Verification items for this drawing (mm, ordinates from the low corner). A direction names the side the tool comes from. Round coordinates to 2 decimals unless told otherwise and drop trailing zeros. Loops run counter-clockwise (first coordinate to the right, second up) from the corner with the lowest first, then second, coordinate; pieces in that order, holes last. Notation, with made-up numbers: (70, 27) - (101, 27) arc R7 ccw to (101, 40) - close; hole circle Ø5 at (71, 12.25). An arc over 180 degrees is marked (long way). Put each result on its own line as item: value.
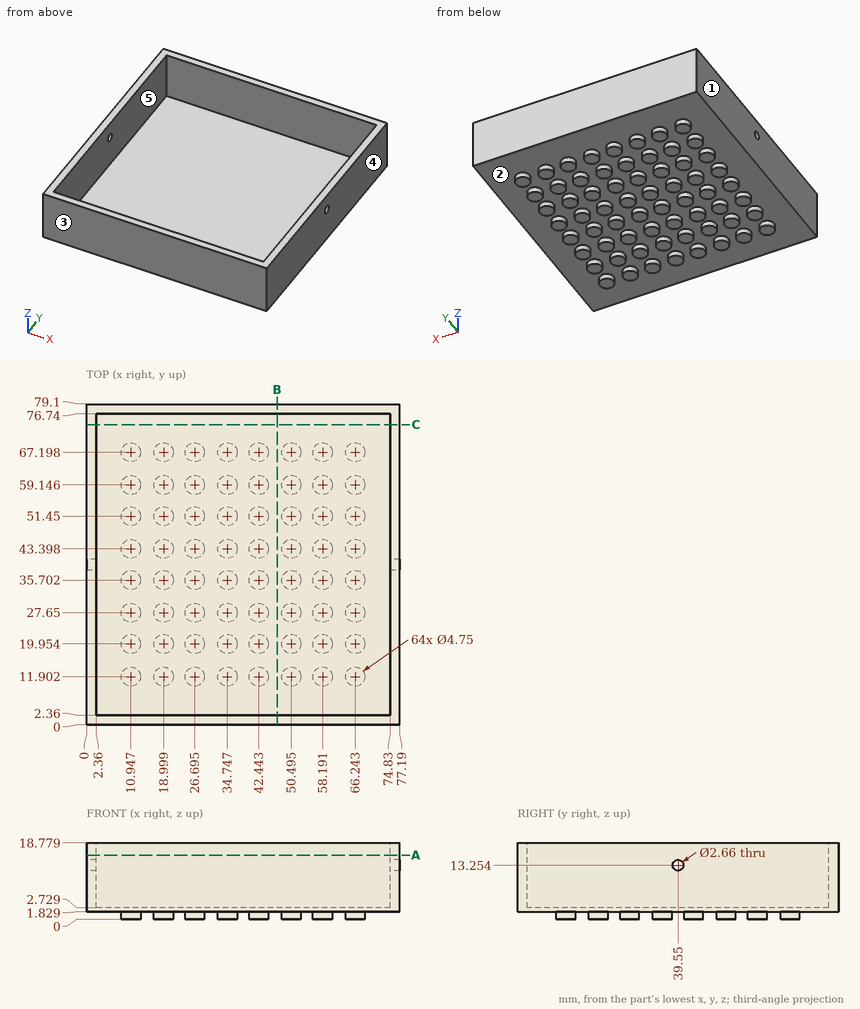
Item 1: Thickness scan on line 1 (Y direction, x = 28.5, z = 16); line 2 (X direction, y = 12, z = 3.75); line 3 (Z direction, x = 14, y = 11.5). Record the ranges inside material, lowest first. Write a range as from..to.
Filled sheet:
line 1: 0..2.36, 76.74..79.1
line 2: 0..2.36, 74.83..77.19
line 3: 1.83..2.73
Item 2: Section check B-B on x = 47. Enter the section's corners in (y, z).
Filled sheet:
outline: (0, 1.83) - (79.1, 1.83) - (79.1, 18.78) - (76.74, 18.78) - (76.74, 2.73) - (2.36, 2.73) - (2.36, 18.78) - (0, 18.78) - close
Item 3: Tool access check on the marked faces 4 and 5. Record the directions out of +Z, -Z, +X, -X, +Y, -Y that give a thin tool (end or side, any length) a straight path to the whole face; none if there is none.
Filled sheet:
face 4: +Z, -Z, +X, +Y, -Y
face 5: +Z
Item 4: Section check C-C on y = 74. Enter the section's corners in (x, z).
Filled sheet:
outline: (0, 1.83) - (77.19, 1.83) - (77.19, 18.78) - (74.83, 18.78) - (74.83, 2.73) - (2.36, 2.73) - (2.36, 18.78) - (0, 18.78) - close
Item 5: Release check for a two-part mould opening along Y. For the marked faces 1, 2 and 3 record: +Y half, -Y half, draft (parallel to the pull), parting line (faces both ways), or undercut.
Filled sheet:
face 1: draft
face 2: undercut
face 3: -Y half
Item 6: Go/stop test with flat-tipped pins: pin 1 (1.5 mm diameter, centred on x = 41, y = 31, fed in from +Z); pin 2 (1 mm diameter, centred on x = 37.5, y = 52.5, fed in from -Z). Record where each tip stops, or that it passes through.
Filled sheet:
pin 1: z = 2.73
pin 2: z = 1.83
Item 7: Section check A-A on z = 15.75. Enter the section's corners in (x, y).
Filled sheet:
outline: (0, 0) - (77.19, 0) - (77.19, 79.1) - (0, 79.1) - close; hole (2.36, 2.36) - (74.83, 2.36) - (74.83, 76.74) - (2.36, 76.74) - close
